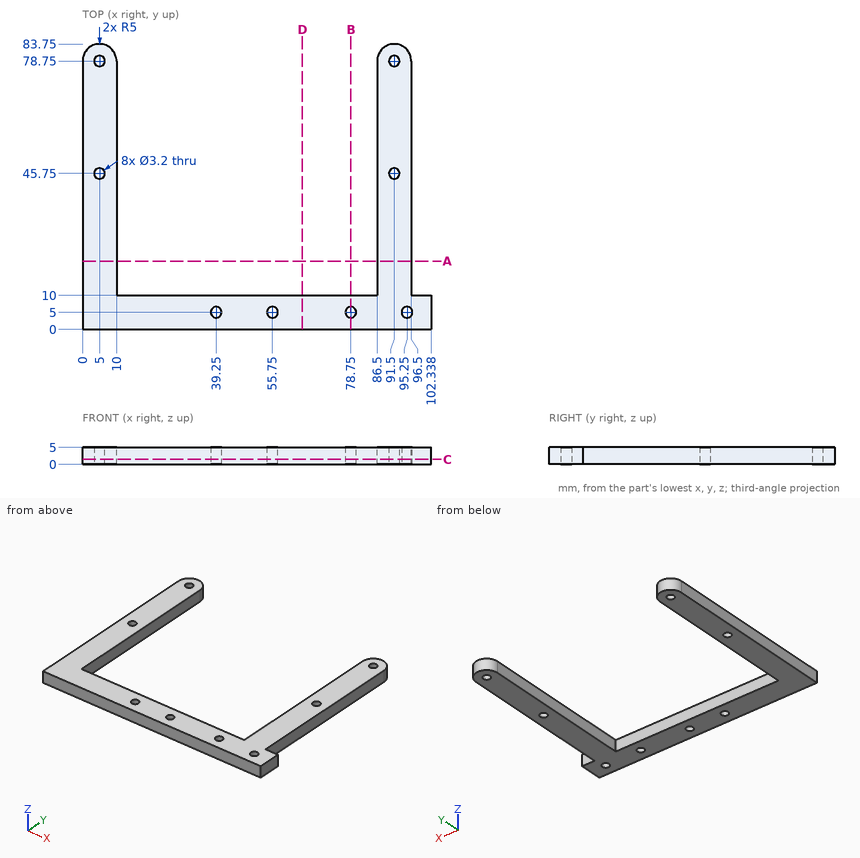
Input: dimensioned drawing with shaded views. Units: mm. Origin: part minimum x, y, z. Give positions to 0.01 mm unless a question says otherwise; leave off trailing zeros. Write each loop counter-clockwise with the first axis right and the second up, starting at its lowest first coordinate (ties: lowest second). Pieces come first, ordered by that corner, then holes. Notation, with made-up numbers: M 17,-26 L 70,-26 A22 cw 70,-16 Z; hole C 55.5,-18.75 d1. An arc over 180 degrees is marked long. Write item = value, one per line. Start each with the question number.
1) Cut plane D-D on x = 64.5. Return the cut outline in (y, z), then the cut area to 3 significant figures.
2) Material intervals for line 1 along X through (y, z) = (5, 2.05); line 2 along Y through (x, z) = (5, 4.1); line 3 along X through (y, z) = (45.75, 3.3), sorted ascending. Write a range as [from, to].
3) Cut plane B-B on x = 78.75. Return the cut outline in (y, z), then the cut area to 3 significant figures.
4) First-contact query: pin 1 Ø4 at (x, y) = (91.5, 78.75) entering from -Z; pin 2 Ø1.5 at (y, z) = (51, 1.5) entering from +X; pin 3 Ø1 at (x, z) = (27.5, 1.5) entering from +Y. Flat tips, straight axial feed; report the tip coordinate or a pass-through.
5) Cut plane A-A on y = 20. Return the cut outline in (x, z), then the cut area to 3 significant figures.
6) Cut plane C-C on z = 1.5. Count the separate pieces of the cut face and the enclosed holes in it, then the cut area to 3 significant figures.
Solved:
q1.outline = M 0,0 L 10,0 L 10,5 L 0,5 Z
q1.area = 50.0 mm2
q2.line_1 = [0, 37.65], [40.85, 54.15], [57.35, 77.15], [80.35, 93.65], [96.85, 102.34]
q2.line_2 = [0, 44.15], [47.35, 77.15], [80.35, 83.75]
q2.line_3 = [0, 3.4], [6.6, 10], [86.5, 89.9], [93.1, 96.5]
q3.outline = M 0,0 L 3.4,0 L 3.4,5 L 0,5 Z; M 6.6,0 L 10,0 L 10,5 L 6.6,5 Z
q3.area = 34.0 mm2
q4.pin_1 = 0
q4.pin_2 = 96.5
q4.pin_3 = 10
q5.outline = M 0,0 L 10,0 L 10,5 L 0,5 Z; M 86.5,0 L 96.5,0 L 96.5,5 L 86.5,5 Z
q5.area = 100 mm2
q6.separate_pieces = 1
q6.enclosed_holes = 8
q6.area = 2,410 mm2
